```python
from build123d import *

# Parameters (mm, degrees)
F0_W        = 7.6837688684
F0_H        = 17.6492575556
F1_DEPTH    = 31.75
F0_W_2      = 101.6
F0_H_2      = 50.4952
F2_DEPTH    = 25.4
F3_T1_DEPTH = 43.0492575556


# Not quite as in the source:
# - a fillet or chamfer that OpenCascade refuses, or shapes differently, is made with other operations: its cross-section is extruded or revolved along the edge and cut away or added


with BuildPart() as f1:
    # F0 (on Front) → F1 (new body)
    with BuildSketch(Plane.XZ):
        with Locations((38.4069420397, 0)):
            Rectangle(F0_W, F0_H)
    extrude(amount=F1_DEPTH)

    # F0 (on Front) → F2 (join)
    with BuildSketch(Plane.XZ):
        Rectangle(F0_W_2, F0_H_2)
        with Locations((38.4069420397, 0)):
            Rectangle(F0_W, F0_H, mode=Mode.SUBTRACT)
    extrude(amount=F2_DEPTH)

    # F3: fillet of radius 5.08 on 2 edges, made by hand

    # F3_s2 → F3_t1 (cut)
    with BuildSketch(Plane.XY.offset(-21.5246287778)):
        with BuildLine():
            ThreePointArc((42.248826474, -26.67), (40.7609289224, -30.2621024484), (37.168826474, -31.75))
            Line((37.168826474, -31.75), (42.248826474, -31.75))
            Line((42.248826474, -31.75), (42.248826474, -26.67))
        make_face()
        with BuildLine():
            ThreePointArc((39.6450576055, -31.75), (36.0529551571, -30.2621024484), (34.5650576055, -26.67))
            Line((34.5650576055, -26.67), (34.5650576055, -31.75))
            Line((34.5650576055, -31.75), (39.6450576055, -31.75))
        make_face()
    extrude(amount=F3_T1_DEPTH, mode=Mode.SUBTRACT)


solid = f1.part
```
Model file for the job. Use its own axes, mm. A direction names the side the tool comes from. Round coordinates to 2 decimals unless told otherwise and drop trailing zeros. Order: outer loops, then holes, each group sorted by start corner. A loop starts at its lowest first (then second) coordinate and runs counter-clockwise, first axis right, second up. Notation, with made-up numbers: M 43,26.5 L 84,26.5 A17 cw 84,51.5 Z; hole C 49,-20.5 d7. An arc over 180 degrees is marked long. Use CSV: the item, a comma, the result in double quotes.
Item 1: Pin check, flat tips, straight feed: pin 1 (0.6 mm diameter, centred on y = -26, z = -2.5, fed in from -X); pin 2 (5 mm diameter, centred on x = 39, y = -28, fed in from +Z); pin 3 (15 mm diameter, centred on x = 15.5, z = -12, fed in from -Y). Stop position of each tip, or through.
Worked answers:
pin 1,"x = 34.57"
pin 2,"z = 8.82"
pin 3,"y = -25.4"
Item 2: Saw through at B-B (x = -17.5). List the corners of the cut face in (y, z).
Worked answers:
outline,"M -25.4,-25.25 L 0,-25.25 L 0,25.25 L -25.4,25.25 Z"
Item 3: Saw through at A-A (z = 2). List the corners of the cut face in (x, y).
Worked answers:
outline,"M -50.8,-25.4 L 34.57,-25.4 L 34.57,-26.67 A5.08 ccw 38.41,-31.6 A5.08 ccw 42.25,-26.67 L 42.25,-25.4 L 50.8,-25.4 L 50.8,0 L -50.8,0 Z"
Item 4: Which spindle directions (+Z, -Z, +X, -X, +Y, -Y) get a long thin tool onto all of the face, cutting with end or side? Do faces 1 (the face through (38, -28, 8.825)), 2 (the face through (38, -28, -8.825)), 3 (the face through (50.8, -13, 0)). Say none if no direction does.
Worked answers:
face 1,"+Z, +X, -X, -Y"
face 2,"-Z, +X, -X, -Y"
face 3,"+Z, -Z, +X, +Y, -Y"
Item 5: Probe probe 1 along Y at (x, z) = (13, -22); probe 2 along X at (y, z) = (-26.5, 2); probe 3 along X at (y, z) = (-28.5, 4). List the from-to ranges inside material, lowest first.
Worked answers:
probe 1,"-25.4 to 0"
probe 2,"34.57 to 42.25"
probe 3,"34.91 to 41.91"
Item 6: Saw through at C-C (z = 21.5). List the corners of the cut face in (x, y), plus the area to 3 significant figures.
Worked answers:
outline,"M -50.8,-25.4 L 50.8,-25.4 L 50.8,0 L -50.8,0 Z"
area,"2,580 mm²"
